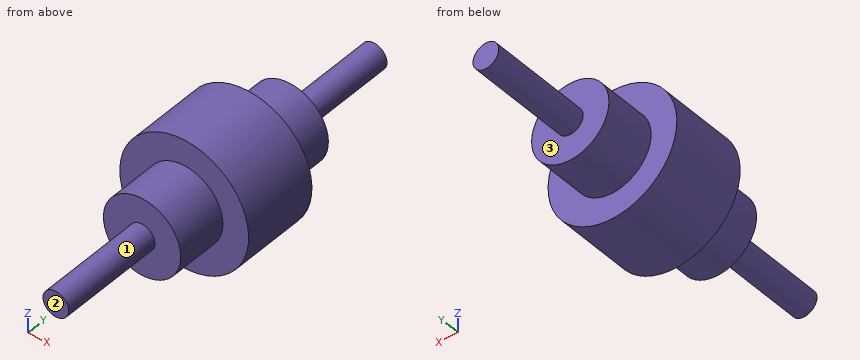
```python
from build123d import *


with BuildPart() as part:
    # Sketch1 → Revolve1 (revolve)
    with BuildSketch(Plane.XY, mode=Mode.PRIVATE) as revolve1_sk:
        Polygon((0, 0), (10, 0), (10, 1.693933425), (10, 81.693933425), (30, 81.693933425), (30, 121.693933425), (50, 121.693933425), (50, 181.693933425), (30, 181.693933425), (30, 221.693933425), (10, 221.693933425), (10, 301.693933425), (0, 301.693933425), align=None)
    revolve(revolve1_sk.sketch.rotate(Axis((0, 99.4903565, 0), (0, -1, 0)), 90), axis=Axis((0, 99.4903565, 0), (0, -1, 0)))  # turned: the seam where the file's is


solid = part.part
```
Work out the finished part from the listing and answer in its coordinate system (mm). Face numbers are marked on the shaded views. A direction names the side the tool comes from. Round coordinates to 2 decimals unless told otherwise and drop trailing zeros. Write each loop counter-clockwise with the first axis right and the second up, starting at its lowest first coordinate (ties: lowest second). Pieces come first, ordered by that corner, then holes.
1) Consider probe 1 along Y at (x, z) = (11, -44.5); probe 2 along Y at (x, z) = (-19, 0.5); probe 3 along Z at (x, y) = (-3.5, 268.5). Determine where each line is inside the solid, lowest interval first.
2) A cutting plane is placed at B-B on z = 0. Determine the outline of the cut face in (x, y), and give its area (3 significant figures).
3) Which of the six approach directions +Z, -Z, +X, -X, +Y, -Y give full straight-line access (tool end or side, diameter ignored) to the marked faces 1, 2 and 3?
4) A cutting plane is placed at C-C on y = 158.5. Determine the outline of the cut face in (x, z), and give its area (3 significant figures).
5) A cutting plane is placed at D-D on z = 25.5. Determine the outline of the cut face in (x, y), and give its area (3 significant figures).
6) A cutting plane is placed at A-A on x = 0. Determine the outline of the cut face in (y, z).
7) Flat-ended cylindrical pins translate along their axes: P1, Ø5, axis at x = 26, y = 136, coming from the -Z side; P2, Ø1.5, axis at y = 103, z = -27, coming from the -X side; P3, Ø12, axis at x = 26, z = -27.5, coming from the -Y side. Find the tip coordinate at first contact, or state that the pin passes through.
Entries:
1. probe 1: y = 121.69 to 181.69
1. probe 2: y = 81.69 to 221.69
1. probe 3: z = -9.37 to 9.37
2. outline: (-50, 121.69) - (-30, 121.69) - (-30, 81.69) - (-10, 81.69) - (-10, 0) - (10, 0) - (10, 81.69) - (30, 81.69) - (30, 121.69) - (50, 121.69) - (50, 181.69) - (30, 181.69) - (30, 221.69) - (10, 221.69) - (10, 301.69) - (-10, 301.69) - (-10, 221.69) - (-30, 221.69) - (-30, 181.69) - (-50, 181.69) - close
2. area: 14,000 mm2
3. face 1: -Y
3. face 2: +Z, -Z, +X, -X, -Y
3. face 3: +Y
4. outline: circle Ø100 at (0, 0)
4. area: 7,850 mm2
5. outline: (-43.01, 121.69) - (-15.8, 121.69) - (-15.8, 81.69) - (15.8, 81.69) - (15.8, 121.69) - (43.01, 121.69) - (43.01, 181.69) - (15.8, 181.69) - (15.8, 221.69) - (-15.8, 221.69) - (-15.8, 181.69) - (-43.01, 181.69) - close
5. area: 7,690 mm2
6. outline: (0, -10) - (81.69, -10) - (81.69, -30) - (121.69, -30) - (121.69, -50) - (181.69, -50) - (181.69, -30) - (221.69, -30) - (221.69, -10) - (301.69, -10) - (301.69, 10) - (221.69, 10) - (221.69, 30) - (181.69, 30) - (181.69, 50) - (121.69, 50) - (121.69, 30) - (81.69, 30) - (81.69, 10) - (0, 10) - close
7. P1: stops at z = -44.13
7. P2: stops at x = -14.52
7. P3: stops at y = 121.69
